For this review, use the dimensioned drawing (mm, ordinates from the lowest corner) and the shaded views. A direction names the side the tool comes from. Round coordinates to 2 decimals unless told otherwise and drop trailing zeros. Write each loop counter-clockwise with the first axis right and the second up, starting at its lowest first coordinate (ties: lowest second). Pieces come first, ordered by that corner, then holes. Notation, with made-up numbers: M -29.5,-17.5 L -24.5,-17.5 A20 ccw -24.5,10.5 Z; hole C 27.5,68.5 d11. An arc over 180 degrees is marked long. Answer in a Markdown table with one row per item.
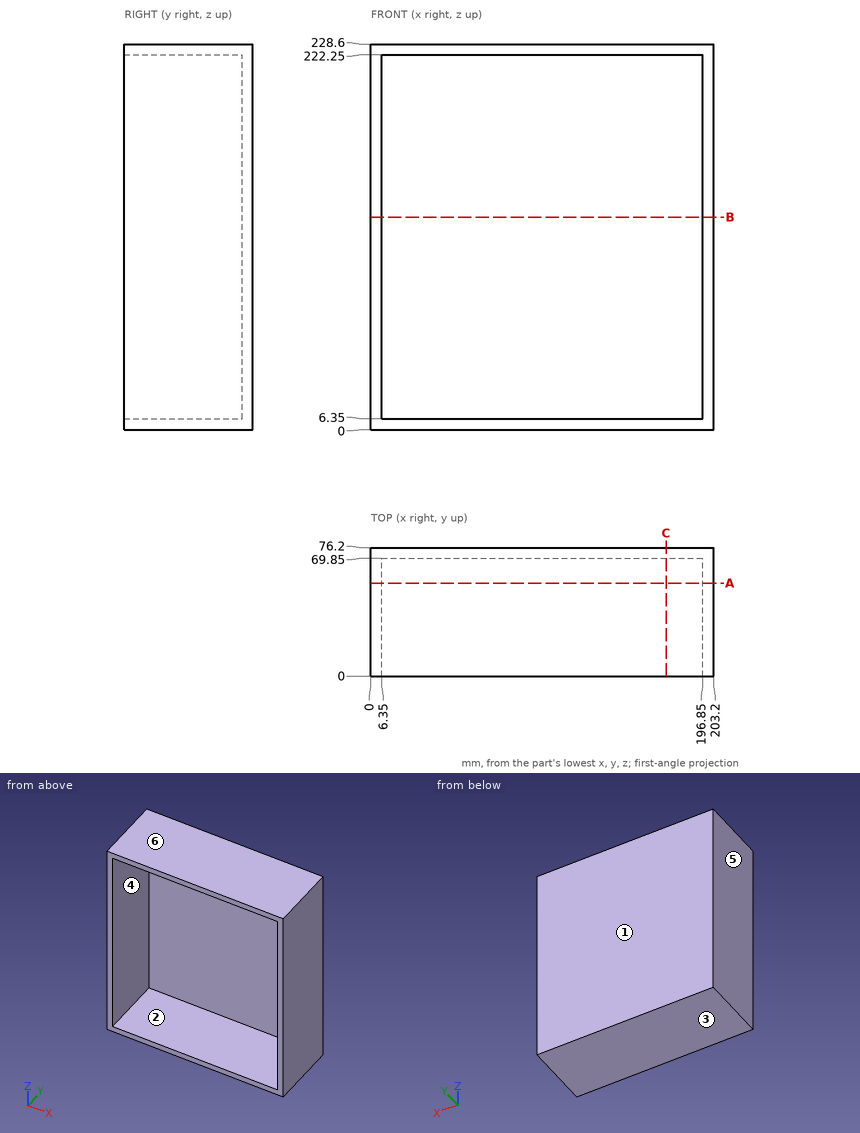
Q1. Take a section at B-B (z = 126). State the section outline as (x, y) points, then the cut area to 3 significant figures.
Found:
| item | result |
|---|---|
| outline | M 0,0 L 6.35,0 L 6.35,69.85 L 196.85,69.85 L 196.85,0 L 203.2,0 L 203.2,76.2 L 0,76.2 Z |
| area | 2,180 mm² |
Q2. Machinability: for the marked faces 1 and 2, which of the approach directions +Z, -Z, +X, -X, +Y, -Y give a long, thin tool a straight path to every point of the face, cutting with its end or side? Answer none if there is none.
Found:
| item | result |
|---|---|
| face 1 | +Z, -Z, +X, -X, +Y |
| face 2 | -Y |
Q3. Mouldability with a two-part tool opening along Z and no side actions: class the marked faces 3, 4, 5 and 6 as +Z half, -Z half, draft (parallel to the pull), parting line (faces both ways), or undercut.
Found:
| item | result |
|---|---|
| face 3 | -Z half |
| face 4 | undercut |
| face 5 | draft |
| face 6 | +Z half |
Q4. For probe 1 along X at (y, z) = (68.5, 16); probe 2 along Z at (x, y) = (74.5, 8); probe 3 along Y at (x, z) = (89, 98), list the stretches that pass through material, from the lowest coordinate up.
Found:
| item | result |
|---|---|
| probe 1 | 0 to 6.35, 196.85 to 203.2 |
| probe 2 | 0 to 6.35, 222.25 to 228.6 |
| probe 3 | 69.85 to 76.2 |
Q5. Take a section at A-A (y = 55). State the section outline as (x, z) points.
Found:
| item | result |
|---|---|
| outline | M 0,0 L 203.2,0 L 203.2,228.6 L 0,228.6 Z; hole M 6.35,6.35 L 196.85,6.35 L 196.85,222.25 L 6.35,222.25 Z |
Q6. Take a section at C-C (x = 175). State the section outline as (y, z) points, then the cut area to 3 significant figures.
Found:
| item | result |
|---|---|
| outline | M 0,0 L 76.2,0 L 76.2,228.6 L 0,228.6 L 0,222.25 L 69.85,222.25 L 69.85,6.35 L 0,6.35 Z |
| area | 2,340 mm² |
Q7. Insertion check: P1, Ø12, axis at x = 131.5, y = 49.5, coming from the -Z side; P2, Ø12, axis at x = 65.5, z = 127.5, coming from the -Y side. Each pin has a flat end and moves straight along its axis. Give the tip position at first contact, or say it passes through.
Found:
| item | result |
|---|---|
| P1 | z = 0 |
| P2 | y = 69.85 |
